from build123d import *


with BuildPart() as f1:
    # F0 (on Front) → F1 (revolve)
    with BuildSketch(Plane.XZ):
        Polygon((-44, 3), (-41.404769, 3), (-44.119512, 5.589822), (-44, 3.058995), align=None)
        with BuildLine():
            Line((-46.5, 0), (0, 0))
            Line((0, 0), (0, 3))
            Line((0, 3), (-41.404769, 3))
            Line((-41.404769, 3), (-44, 3))
            Line((-44, 3), (-44, 3.058995))
            Line((-44, 3.058995), (-44.119512, 5.589822))
            Line((-44.119512, 5.589822), (-46.5, 56))
            Line((-46.5, 56), (-48.5, 56))
            Line((-48.5, 56), (-48.5, 2))
            ThreePointArc((-48.5, 2), (-47.914214, 0.585786), (-46.5, 0))
        make_face()
    revolve(axis=Axis((0, 0, 1.5), (0, 0, -1)))


solid = f1.part
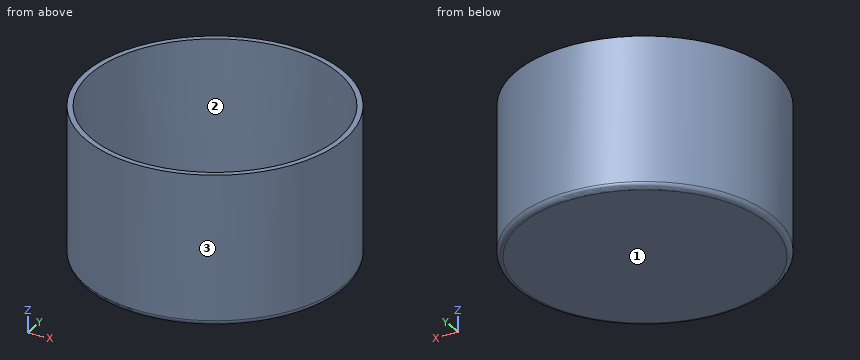
Read the model definition and answer for the solid it produces. Units are mm, in the model's axes. Face numbers are marked on the shaded views. Coordinates: 2 decimals unless noted, no trailing zeros. Loops run counter-clockwise (first coordinate to the right, second up) from the corner with the lowest first, then second, coordinate; pieces in that order, holes last.
Q1. The part is cut by section C-C on z = 17.5. Write down the section's boundary in (x, y), and give its area (3 significant figures).
Q2. The part is cut by section A-A on x = 0. Write down the section's boundary in (y, z), and give its area (3 significant figures).
Q3. The mould has two halves that part along Y. Classify the marked faces 1, 2 and 3: +Y half, -Y half, draft (parallel to the pull), parting line (faces both ways), or undercut.
Q4. The part is cut by section D-D on z = 33. Write down the section's boundary in (x, y).
Q5. Each of these flat-tipped pins is pushed along its axis until it touches: pin 1 Ø5 at (y, z) = (-10.5, 43) entering from +X; pin 2 Ø1.5 at (y, z) = (-2, 30.5) entering from -X; pin 3 Ø3 at (x, z) = (-17.5, 43) entering from -Y. Where does it stop, or does it pass through?
Q6. Consider probe 1 along Z at (x, y) = (6.5, -12); probe 2 along X at (y, z) = (24, 16); probe 3 along Y at (x, z) = (-28, 8.5). Determine where each line is inside the solid, lowest interval first.
Results below:
1. outline: circle Ø97 at (0, 0); hole circle Ø89.36 at (0, 0)
1. area: 1,120 mm2
2. outline: (-48.5, 2) arc R2 ccw to (-46.5, 0) - (46.5, 0) arc R2 ccw to (48.5, 2) - (48.5, 56) - (46.5, 56) - (44.12, 5.59) - (41.4, 3) - (-41.4, 3) - (-44.12, 5.59) - (-46.5, 56) - (-48.5, 56) - close
2. area: 641 mm2
3. face 1: draft
3. face 2: undercut
3. face 3: parting line
4. outline: circle Ø97 at (0, 0); hole circle Ø90.83 at (0, 0)
5. pin 1: stops at x = 47.84
5. pin 2: stops at x = -48.48
5. pin 3: stops at y = -45.78
6. probe 1: z = 0 to 3
6. probe 2: x = -42.15 to -37.61, 37.61 to 42.15
6. probe 3: y = -39.6 to -34.27, 34.27 to 39.6
